The figure shows three views and two pictorial views of one solid part (mm, origin at its lowest corner). Answer the questions. A direction names the side the tool comes from. Round coordinates to 2 decimals unless told otherwise and drop trailing zeros. Loops run counter-clockwise (first coordinate to the right, second up) from the corner with the lowest first, then second, coordinate; pieces in that order, holes last. Notation, with made-up numbers: (-37.5, -34.5) -> (-22.5, -34.5) arc R29 cw to (-22.5, -9.5) -> close; hole circle Ø11 at (88, 24). An arc over 180 degrees is marked (long way). Use a Markdown table: item, result. Add a question column.
Q1. Which of the six approach directions +Z, -Z, +X, -X, +Y, -Y give full straight-line access (tool end or side, diameter ignored) to the marked faces 1, 2 and 3?
Q2. Section A-A on z = 12 is taken. Give the vertices of the cut face in (x, y).
Q3. Section C-C on x = 7.5 is taken. Give the vertices of the cut face in (y, z).
Q4. For a pull along X with two mould halves and no side action, classify the marked faces 4, 5 and 6 as released by +X, released by -X, zero draft, split by the parting line, or undercut.
Q5. Section D-D on y = 25.5 is taken. Give the vertices of the cut face in (x, z), then the cut area to 3 significant figures.
Q6. Consider line 1 (X direction, y = 6.5, z = 18); line 2 (Z direction, x = 29, y = 10.5); line 3 (Z direction, x = 18, y = 9). Determine where each line is inside the solid, lowest interval first.
Q7. Section B-B on y = 17 is taken. Give the vertices of the cut face in (x, z), then the cut area to 3 significant figures.
Q8. Given pin 1 Ø18 at (x, y) = (20.5, 9.5) entering from +Z; pin 2 Ø6 at (x, y) = (32, 14.5) entering from -Z, each flat-ended and moving along its own axis, determine where each tip first touches the part or whether it passes through.
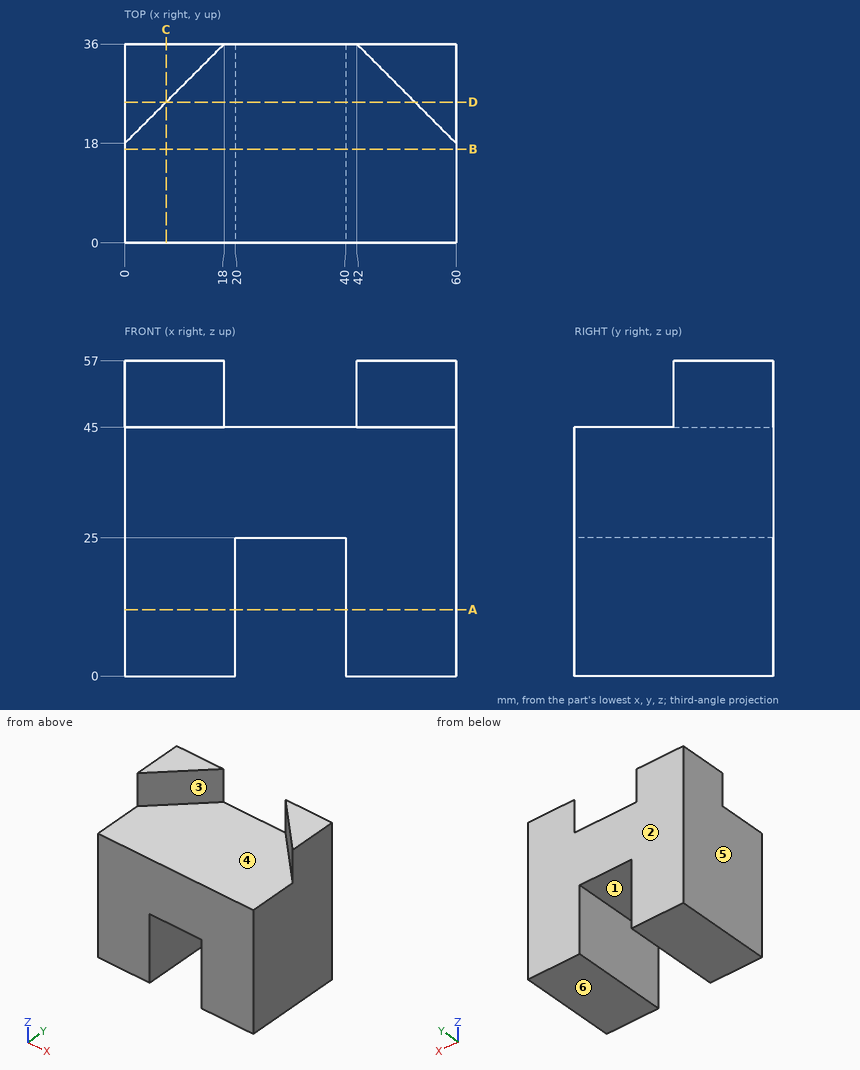
Checked values:
| question | item | result |
|---|---|---|
| 1 | face 1 | -Z, +Y, -Y |
| 1 | face 2 | +Z, -Z, +X, -X, +Y |
| 1 | face 3 | +Z, -Y |
| 2 | outline | (0, 0) -> (20, 0) -> (20, 36) -> (0, 36) -> close; (40, 0) -> (60, 0) -> (60, 36) -> (40, 36) -> close |
| 3 | outline | (0, 0) -> (36, 0) -> (36, 57) -> (25.5, 57) -> (25.5, 45) -> (0, 45) -> close |
| 4 | face 4 | undercut |
| 4 | face 5 | released by -X |
| 4 | face 6 | zero draft |
| 5 | outline | (0, 0) -> (20, 0) -> (20, 25) -> (40, 25) -> (40, 0) -> (60, 0) -> (60, 57) -> (52.5, 57) -> (52.5, 45) -> (7.5, 45) -> (7.5, 57) -> (0, 57) -> close |
| 5 | area | 2,380 mm2 |
| 6 | line 1 | x = 0 to 20, 40 to 60 |
| 6 | line 2 | z = 25 to 45 |
| 6 | line 3 | z = 0 to 45 |
| 7 | outline | (0, 0) -> (20, 0) -> (20, 25) -> (40, 25) -> (40, 0) -> (60, 0) -> (60, 45) -> (0, 45) -> close |
| 7 | area | 2,200 mm2 |
| 8 | pin 1 | stops at z = 45 |
| 8 | pin 2 | stops at z = 25 |
